from build123d import *

# Parameters (mm, degrees)
SKETCH1_W           = 360
SKETCH1_H           = 210
SKETCH1_W_2         = 304
SKETCH1_H_2         = 154
BOSS_EXTRUDE1_DEPTH = 5
SKETCH2_R           = 4
CUT_EXTRUDE1_DEPTH  = 10


with BuildPart() as part:
    # Sketch1 → Boss-Extrude1 (new body)
    with BuildSketch(Plane(origin=(0, 0, 0), x_dir=(1, 0, 0), z_dir=(0, 1, 0))):
        Rectangle(SKETCH1_W, SKETCH1_H)
        Rectangle(SKETCH1_W_2, SKETCH1_H_2, mode=Mode.SUBTRACT)
    extrude(amount=BOSS_EXTRUDE1_DEPTH)

    # Sketch2 → Cut-Extrude1 (cut)
    with BuildSketch(Plane(origin=(0, 5, 0), x_dir=(1, 0, 0), z_dir=(0, 1, 0))):
        with Locations((-160, -85)):
            Circle(SKETCH2_R)
        with Locations((160, -85)):
            Circle(SKETCH2_R)
        with Locations((160, 85)):
            Circle(SKETCH2_R)
        with Locations((-160, 85)):
            Circle(SKETCH2_R)
    extrude(amount=-CUT_EXTRUDE1_DEPTH, mode=Mode.SUBTRACT)


solid = part.part
Here's how the part is built. I have some questions about the finished solid (model axes, mm). Round coordinates to 2 decimals unless told otherwise and drop trailing zeros. Write each loop counter-clockwise with the first axis right and the second up, starting at its lowest first coordinate (ties: lowest second). Pieces come first, ordered by that corner, then holes. Notation, with made-up numbers: (71.5, 72) -> (76.5, 72) arc R19 cw to (76.5, 88) -> close; hole circle Ø4 at (-10, 21). An arc over 180 degrees is marked (long way). One line per item, written item: value.
1) Suppose I cut it at A-A on z = 85. List the corners of the cut face in (x, y) for me, plus the area to 3 significant figures.
Filled sheet:
outline: (-180, 0) -> (-164, 0) -> (-164, 5) -> (-180, 5) -> close; (-156, 0) -> (156, 0) -> (156, 5) -> (-156, 5) -> close; (164, 0) -> (180, 0) -> (180, 5) -> (164, 5) -> close
area: 1,720 mm2
2) Suppose I cut it at C-C on y = 1.4. List the corners of the cut face in (x, z) for me.
Filled sheet:
outline: (-180, -105) -> (180, -105) -> (180, 105) -> (-180, 105) -> close; hole circle Ø8 at (-160, -85); hole circle Ø8 at (-160, 85); hole (-152, -77) -> (152, -77) -> (152, 77) -> (-152, 77) -> close; hole circle Ø8 at (160, -85); hole circle Ø8 at (160, 85)
3) Suppose I cut it at B-B on x = -59. List the corners of the cut face in (y, z) for me.
Filled sheet:
outline: (0, -105) -> (5, -105) -> (5, -77) -> (0, -77) -> close; (0, 77) -> (5, 77) -> (5, 105) -> (0, 105) -> close
4) We'd pull the mould along Z, two halves only. Please class faces 1 (the face through (-3, 5, 92)), 2 (the face through (161.846, 2.535, -81.451)): released by +Z, released by -Z, zero draft, split by the parting line, or undercut.
Filled sheet:
face 1: zero draft
face 2: undercut
5) If I drill on line 1 (X direction, y = 3.8, z = -85); line 2 (Z direction, x = 160, y = 2.7); line 3 (X direction, y = 4.65, z = -57.5), over which ranges is the centre line in solid material (lowest first)? Write a range as [from, to].
Filled sheet:
line 1: x = [-180, -164], [-156, 156], [164, 180]
line 2: z = [-105, -89], [-81, 81], [89, 105]
line 3: x = [-180, -152], [152, 180]
6) Suppose I cut it at D-D on z = 57. List the corners of the cut face in (x, y) for me, plus the area to 3 significant figures.
Filled sheet:
outline: (-180, 0) -> (-152, 0) -> (-152, 5) -> (-180, 5) -> close; (152, 0) -> (180, 0) -> (180, 5) -> (152, 5) -> close
area: 280 mm2
